Check sheet for the modelled part. Datum: model origin and axes. Units: mm. A direction names the side the tool comes from. Give positions to 0.01 mm unless a question says otherwise; leave off trailing zeros. Order: outer loops, then holes, each group sorted by start corner. A loop starts at its lowest first (then second) coordinate and runs counter-clockwise, first axis right, second up. Notation, with made-up numbers: M 28.25,79 L 64.25,79 A13 ccw 64.25,99 Z; hole C 33.25,58.5 d1. An arc over 180 degrees is marked long. Answer in a Markdown table with one row per item. Add a question column.
Autodesk Inventor part; units mm, degrees
ref_plane "Work Plane1" through (0, 7.5, 0) normal (0, 1, 0) x (-1, 0, 0)
ref_plane "YZ Plane" through (0, 0, 0) normal (1, 0, 0) x (0, 1, 0)
ref_plane "XY Plane" through (0, 0, 0) normal (0, 0, 1) x (1, 0, 0)
sketch "Sketch1" plane through (0, 0, 0) normal (0, 0, 1) x (1, 0, 0)
  circle A0 centre (0, 0) radius 4.45
  circle A1 centre (0, 0) radius 7.5
  dimension "d0" = 8.9
  dimension "d1" = 15
extrude "Extrusion1" add sketch "Sketch1" along normal blind 60
ref_plane "Work Plane1" through (0, 7.5, 0) normal (0, 1, 0) x (-1, 0, 0)
sketch "Sketch2" plane through (0, 7.5, 0) normal (0, 1, 0) x (-1, 0, 0)
  line L0 (2.5, 45) -> (-2.5, 45)
  line L1 (-2.5, 45) -> (-2.5, 0)
  line L2 (-2.5, 0) -> (2.5, 0)
  line L3 (2.5, 0) -> (2.5, 45)
  line L4 (7.5, 60) -> (-7.5, 60)
  line L5 (-7.5, 0) -> (7.5, 0)
  point P0 (0, 0)
  dimension "d4" = 45
  dimension "d6" = 5
  dimension "d7" = 2.5
  dimension "d22" = 0
extrude "Extrusion2" cut sketch "Sketch2" against normal through all
sketch "Sketch3" plane through (0, 0, 60) normal (0, 0, 1) x (1, 0, 0)
  circle A0 centre (0, 0) radius 3.2
  circle A1 centre (0, 0) radius 4.45
  dimension "d10" = 6.4
extrude "Extrusion3" add sketch "Sketch3" against normal blind 10
sketch "Sketch4" plane through (0, 0, 0) normal (0, 0, -1) x (-1, 0, 0)
  circle A0 centre (0, 0) radius 4.45
extrude "Extrusion4" add sketch "Sketch4" against normal blind 5
sketch "Sketch5" plane through (0, 0, 0) normal (0, 0, -1) x (0, -1, 0)
  line L0 (-5, -5) -> (5, -5)
  line L1 (5, -5) -> (5, 5)
  line L2 (5, 5) -> (-5, 5)
  line L3 (-5, 5) -> (-5, -5)
  point P0 (0, 0)
  dimension "d16" = 10
  dimension "d17" = 5
  dimension "d18" = 10
  dimension "d19" = 5
extrude "Extrusion5" cut sketch "Sketch5" against normal blind 5
properties part number "Rotation"
Q1. Cross-section at C-C (z = 14.5). Record the boundary of the cut face in (x, y).
Q2. Draft check along X on faces 1 (the flat face through (2, -3, 60)), 2 (the cylindrical face through (7.154, -2.253, 29.58)), 3 (the flat face through (-5, 0, 2)). Enter one of: pulls with the +X half, pulls with the -X half, needs draft (parallel to the pull), parting line crosses it, or undercut.
Q3. Tool access check on faces 4 (the cylindrical face through (-4.446, -0.196, 27.185)), 5 (the flat face through (-2.5, -5, 22)), 6 (the cylindrical face through (-2.539, -1.947, 55.07)). Record the directions out of +Z, -Z, +X, -X, +Y, -Y that give a thin tool (end or side, any length) a straight path to the whole face; none if there is none.
Q4. Cross-section at B-B (x = 0). Record the boundary of the cut face in (y, z), and give its area (4 significant figures).
Q5. Thickness scan on probe 1 along Y at (x, z) = (0, 56); probe 2 along X at (y, z) = (0, 37); probe 3 along Z at (x, y) = (-2.5, -2.5). Record the ranges inside material, lowest first.
Q6. Cross-section at D-D (x = 6). Record the boundary of the cut face in (y, z), and give its area (3 significant figures).
Q7. Go/stop test with flat-tipped pins: pin 1 (1.2 mm diameter, centred on x = -4, z = 1.5, fed in from -Y); pin 2 (3 mm diameter, centred on x = 3, z = 1.5, fed in from +Y); pin 3 (3 mm diameter, centred on x = 0.5, y = 3, fed in from -Z). Record where each tip stops, or that it passes through.
Q8. Cross-section at A-A (y = 0). Record the boundary of the cut face in (x, z), and give its area (4 significant figures).
Values follow:
| question | item | result |
|---|---|---|
| 1 | outline | M -2.5,-7.07 L -2.5,-3.68 A4.45 cw -2.5,3.68 L -2.5,7.07 A7.5 ccw Z; M 2.5,-7.07 A7.5 ccw 2.5,7.07 L 2.5,3.68 A4.45 cw 2.5,-3.68 Z |
| 2 | face 1 | needs draft |
| 2 | face 2 | parting line crosses it |
| 2 | face 3 | undercut |
| 3 | face 4 | -Z |
| 3 | face 5 | -Z, +Y, -Y |
| 3 | face 6 | +Z, -Z |
| 4 | outline | M -7.5,45 L -4.45,45 L -4.45,50 L -3.2,50 L -3.2,60 L -7.5,60 Z; M 3.2,50 L 4.45,50 L 4.45,45 L 7.5,45 L 7.5,60 L 3.2,60 Z |
| 4 | area | 116.5 mm² |
| 5 | probe 1 | -7.5 to -3.2, 3.2 to 7.5 |
| 5 | probe 2 | -7.5 to -4.45, 4.45 to 7.5 |
| 5 | probe 3 | 50 to 60 |
| 6 | outline | M -4.5,0 L 4.5,0 L 4.5,60 L -4.5,60 Z |
| 6 | area | 540 mm² |
| 7 | pin 1 | y = -6.69 |
| 7 | pin 2 | y = 7.07 |
| 7 | pin 3 | z = 45 |
| 8 | outline | M -7.5,0 L -5,0 L -5,5 L -4.45,5 L -4.45,50 L -3.2,50 L -3.2,60 L -7.5,60 Z; M 3.2,50 L 4.45,50 L 4.45,5 L 5,5 L 5,0 L 7.5,0 L 7.5,60 L 3.2,60 Z |
| 8 | area | 385.5 mm² |
